from build123d import *

# Parameters (mm, degrees)
PAD_DEPTH       = 155
SKETCH001_R     = 1.5
SKETCH001_W     = 13
SKETCH001_H     = 130
POCKET_DEPTH    = 12.001
SKETCH002_W     = 5.583172
SKETCH002_H     = 23.950112
POCKET001_DEPTH = 155.001
SKETCH003_W     = 22
SKETCH003_H     = 24
POCKET002_DEPTH = 12.001
SKETCH004_W     = 11.5
SKETCH004_H     = 12.924639
POCKET003_DEPTH = 31
SKETCH005_W     = 12
SKETCH005_H     = 25
PAD001_DEPTH    = 10
SKETCH006_R     = 1.35
POCKET004_DEPTH = 155.001
SKETCH007_R     = 1.5
POCKET005_DEPTH = 12.001003


with BuildPart() as part:
    # Sketch → Pad (new body)
    with BuildSketch(Plane.XY):
        with BuildLine():
            Line((39.5, 4.836187), (-20, 4.836187))
            Line((-20, 4.836187), (-20, -7.163813))
            ThreePointArc((20, -7.163813), (0, 0), (-20, -7.163813))
            Line((20, -7.163813), (39.5, -7.163813))
            Line((39.5, 4.836187), (39.5, -7.163813))
        make_face()
    extrude(amount=-PAD_DEPTH)

    # Sketch001 → Pocket (cut, through all)
    with BuildSketch(Plane.XZ.offset(7.163813)):
        with Locations((28.5, -135)):
            Circle(SKETCH001_R)
        with Locations((34.5, -135)):
            Circle(SKETCH001_R)
        with Locations((33, -65)):
            Rectangle(SKETCH001_W, SKETCH001_H)
    extrude(amount=-POCKET_DEPTH, mode=Mode.SUBTRACT)

    # Sketch002 → Pocket001 (cut, through all)
    with BuildSketch(Plane(origin=(0, 0, -155), x_dir=(1, 0, 0), z_dir=(0, 0, -1))):
        with Locations((-19.791586, -0.240771)):
            Rectangle(SKETCH002_W, SKETCH002_H)
    extrude(amount=-POCKET001_DEPTH, mode=Mode.SUBTRACT)

    # Sketch003 → Pocket002 (cut, through all)
    with BuildSketch(Plane(origin=(0, 4.836187, 0), x_dir=(-1, 0, 0), z_dir=(0, 1, 0))):
        with Locations((6, -42.7)):
            Rectangle(SKETCH003_W, SKETCH003_H)
    extrude(amount=-POCKET002_DEPTH, mode=Mode.SUBTRACT)

    # Sketch004 → Pocket003 (cut)
    with BuildSketch(Plane.XY):
        with Locations((-11.25, 0.936987)):
            Rectangle(SKETCH004_W, SKETCH004_H)
    extrude(amount=-POCKET003_DEPTH, mode=Mode.SUBTRACT)

    # Sketch005 → Pad001 (new body)
    with BuildSketch(Plane.YZ.offset(39.5)):
        with Locations((-1.16381, -142.5)):
            Rectangle(SKETCH005_W, SKETCH005_H)
    extrude(amount=PAD001_DEPTH)

    # Sketch006 → Pocket004 (cut, through all)
    with BuildSketch(Plane(origin=(0, 0, -155), x_dir=(1, 0, 0), z_dir=(0, 0, -1))):
        with Locations((39.5, 1.16381)):
            Circle(SKETCH006_R)
    extrude(amount=-POCKET004_DEPTH, mode=Mode.SUBTRACT)

    # Sketch007 → Pocket005 (cut, through all)
    with BuildSketch(Plane(origin=(0, 4.83619, 0), x_dir=(-1, 0, 0), z_dir=(0, 1, 0))):
        with Locations((-45.5, -135)):
            Circle(SKETCH007_R)
        with Locations((-45.5, -150)):
            Circle(SKETCH007_R)
        with Locations((-33.5, -150)):
            Circle(SKETCH007_R)
        with Locations((-27.5, -150)):
            Circle(SKETCH007_R)
    extrude(amount=-POCKET005_DEPTH, mode=Mode.SUBTRACT)


solid = part.part
Could you check a few things on this model? Use its own coordinates, in mm. A direction names the side the tool comes from. Give positions to 0.01 mm unless a question says otherwise; leave off trailing zeros. Loops run counter-clockwise (first coordinate to the right, second up) from the corner with the lowest first, then second, coordinate; pieces in that order, holes last. Notation, with made-up numbers: (27.25, 44.25) -> (49.25, 44.25) arc R18 ccw to (49.25, 64.25) -> close; hole circle Ø9 at (-39, -4.75). An arc over 180 degrees is marked (long way). Return JSON: item names as keys, results as strings.
Item 1: If we section it at C-C on z = -135: Count the separate pieces of the cut face and the enclosed holes in it, plus the area to 3 significant figures.
Geometry results:
{"separate pieces": "4", "enclosed holes": "1", "area": "492 mm²"}
Item 2: If we section it at D-D on z = -36.5: List the corners of the cut face in (x, y) for me.
Geometry results:
{"outline": "(5, -0.4) arc R31.5 cw to (20, -7.16) -> (26.5, -7.16) -> (26.5, 4.84) -> (5, 4.84) -> close"}
Item 3: I'm going to push flat-ended pins straight in: pin 1 (1.5 mm diameter, centred on y = 1.5, z = -31.5, fed in from +X); pin 2 (3.5 mm diameter, centred on x = 42.5, y = -3, fed in from +Z); pin 3 (10 mm diameter, centred on x = -4, z = -22, fed in from -Y). Where does each tip first touch, or does it pass through?
Geometry results:
{"pin 1": "stops at x = 26.5", "pin 2": "stops at z = -130", "pin 3": "stops at y = -0.48"}
Item 4: I need wall thicknesses on L1, parallel to X at y = 2.25, z = -150; L2, parallel to Z at x = 45.5, y = -4.25; L3, parallel to Z at x = 33.5, y = -3. Which ranges of each line are inside material? Lowest first, please. Write a range as from..to.
Geometry results:
{"L1": "x = -17..26, 29..32, 35..44, 47..49.5", "L2": "z = -155..-151.5, -148.5..-136.5, -133.5..-130", "L3": "z = -155..-151.5, -148.5..-136.12, -133.88..-130"}
Item 5: Which directions (+Z, -Z, +X, -X, +Y, -Y) give clear straight access to the entire face, cutting with the end or side of a thin tool? Please do faces 4 (the flat face through (26.5, -1, -66)), 5 (the flat face through (5, 2, -43)), 6 (the flat face through (25, -7.164, -94)).
Geometry results:
{"face 4": "+Z, +X, +Y, -Y", "face 5": "-X, +Y, -Y", "face 6": "+Z, -Z, +X, -X, -Y"}
Item 6: We'd pull the mould along Y, two halves only. Please class faces 1 (the flat face through (-5.5, 2, -15)), 2 (the flat face through (44, -7.164, -143)), 3 (the cylindrical face through (38.15, -1.22, -142.68)): +Y half, -Y half, draft (parallel to the pull), parting line (faces both ways), or undercut.
Geometry results:
{"face 1": "draft", "face 2": "-Y half", "face 3": "undercut"}
Item 7: If we section it at A-A on y = 2: List the corners of the cut face in (x, z) for me, plus the area to 3 significant figures.
Geometry results:
{"outline": "(-17, -155) -> (49.5, -155) -> (49.5, -130) -> (26.5, -130) -> (26.5, 0) -> (-5.5, 0) -> (-5.5, -30.7) -> (5, -30.7) -> (5, -54.7) -> (-17, -54.7) -> close; hole circle Ø3 at (27.5, -150); hole circle Ø3 at (28.5, -135); hole circle Ø3 at (33.5, -150); hole circle Ø3 at (34.5, -135); hole circle Ø3 at (45.5, -150); hole circle Ø3 at (45.5, -135)", "area": "6,390 mm²"}
Item 8: If we section it at B-B on x = 45.5: List the corners of the cut face in (y, z) for me, plus the area to 3 significant figures.
Geometry results:
{"outline": "(-7.16, -155) -> (4.84, -155) -> (4.84, -151.5) -> (-7.16, -151.5) -> close; (-7.16, -148.5) -> (4.84, -148.5) -> (4.84, -136.5) -> (-7.16, -136.5) -> close; (-7.16, -133.5) -> (4.84, -133.5) -> (4.84, -130) -> (-7.16, -130) -> close", "area": "228 mm²"}
